Geometry check sheet. Reference: drawing and pictorial views, mm from the part's lowest x, y, z. A direction names the side the tool comes from. Give positions to 0.01 mm unless a question says otherwise; leave off trailing zeros. Write each loop counter-clockwise with the first axis right and the second up, starting at its lowest first coordinate (ties: lowest second). Pieces come first, ordered by that corner, then holes.
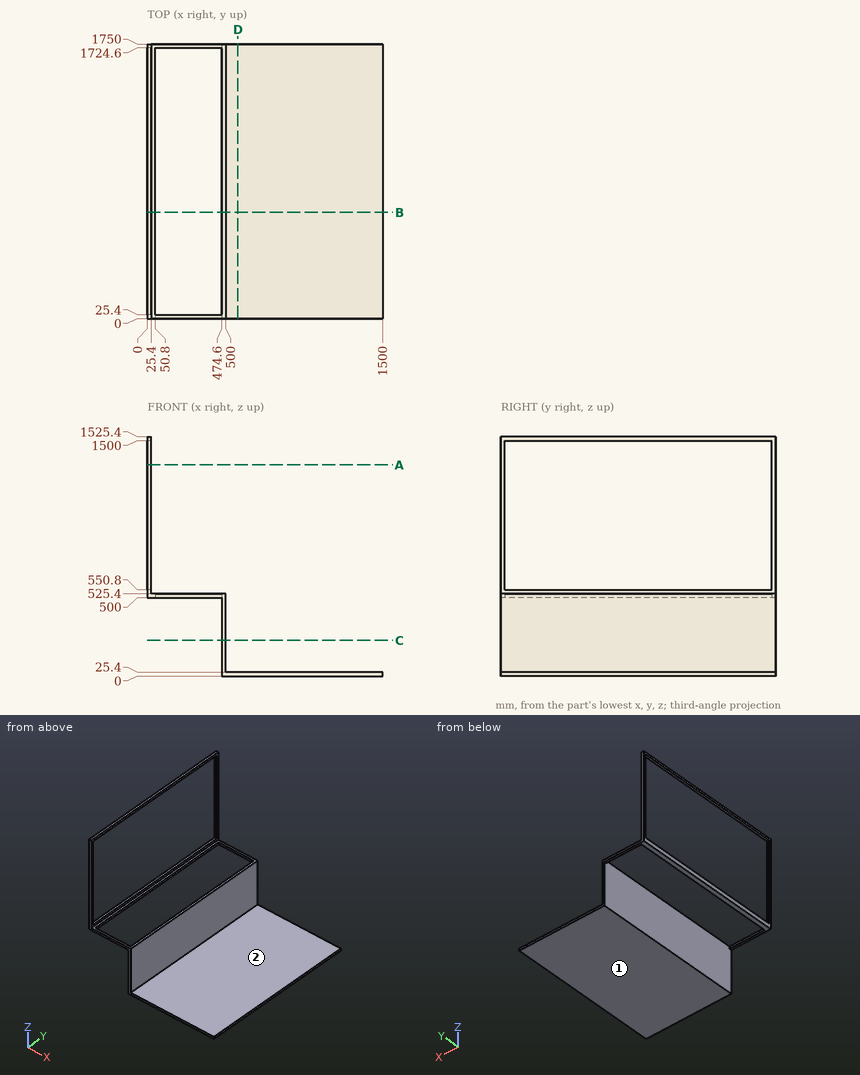
Item 1: Sectioned sample at C-C on z = 227.5. Record the cut outline in (x, y).
Answer key:
outline: (474.6, 0) - (500, 0) - (500, 1750) - (474.6, 1750) - close
Item 2: Sectioned sample at A-A on z = 1345. Record the cut outline in (x, y), then the cut area to 3 significant figures.
Answer key:
outline: (0, 0) - (25.4, 0) - (25.4, 25.4) - (0, 25.4) - close; (0, 1724.6) - (25.4, 1724.6) - (25.4, 1750) - (0, 1750) - close
area: 1,290 mm2
Item 3: Set-up check for the marked faces 1 and 2: record each of +Z, -Z, +X, -X, +Y, -Y from which the full face is reachable in a straight line by a thin tool's end or side.
Answer key:
face 1: -Z, +X, -X, +Y, -Y
face 2: +Z, +X, +Y, -Y
Item 4: Depth check by flat-ended pin: pin 1 (20.5 mm diameter, centred on y = 1070, z = 514, fed in from +X); pin 2 (5 mm diameter, centred on x = 715, y = 335, fed in from +Z); pin 3 (12.5 mm diameter, centred on x = 18.5, y = 1057, fed in from -Z). Enter the tip coordinate at first touch or a pass-through.
Answer key:
pin 1: stops at x = 500
pin 2: stops at z = 25.4
pin 3: stops at z = 500
Item 5: Sectioned sample at D-D on x = 575.5. Record the cut outline in (y, z).
Answer key:
outline: (0, 0) - (1750, 0) - (1750, 25.4) - (0, 25.4) - close
Item 6: Sectioned sample at B-B on y = 677. Record the cut outline in (x, z).
Answer key:
outline: (0, 500) - (50.8, 500) - (50.8, 525.4) - (25.4, 525.4) - (25.4, 550.8) - (0, 550.8) - close; (0, 1500) - (25.4, 1500) - (25.4, 1525.4) - (0, 1525.4) - close; (474.6, 0) - (1500, 0) - (1500, 25.4) - (500, 25.4) - (500, 525.4) - (474.6, 525.4) - close
Item 7: Scan lines: line 1 along Z through (x, y) = (863.5, 819); line 2 along X through (y, z) = (1089, 254.5). Record each from-to range of solid material in increasing order.
Answer key:
line 1: z = 0 to 25.4
line 2: x = 474.6 to 500
